Here's how the part is built. I have some questions about the finished solid (model axes, mm). Face numbers are marked on the shaded views. A direction names the side the tool comes from. Give positions to 0.01 mm unless a question says otherwise; leave off trailing zeros. Answer as CSV lines item,"result". Start each with the question number.
Item 1: Will these pins go through, and if not, where does the flat tip stop? P1, Ø5, axis at x = 19.5, z = 3, coming from the -Y side; P2, Ø6, axis at x = 6.5, z = 2, coming from the -Y side; P3, Ø3, axis at x = 17.5, z = 7.5, coming from the +Y side; P4, Ø6, axis at x = 25, y = 100, coming from the +Z side.
Item 2: If I drill on line 1 along X through (y, z) = (75.5, 7.5); line 2 along X through (y, z) = (86, 7.5); line 3 along Y through (x, z) = (34.5, 7), over which ranges is the centre line in solid material (lowest first)? Write a range as from..to.
Item 3: For the marked faces 3 and 4, which set-ups out of +Z, -Z, +X, -X, +Y, -Y let a thin tool reach every point of the face, with its end or its side?
Item 4: If we mould it in two halves opening along X, with no side actions, what happens to the marked faces 1 and 2? For each: released by +X, released by -X, zero draft, split by the parting line, or undercut.
Item 5: I want a section at A-A on z = 3.75. Give the number of separate pieces and of enclosed holes in the cut face, plus the area to 3 significant figures.
from build123d import *

# Parameters (mm, degrees)
SKETCH1_R           = 5
BOSS_EXTRUDE1_DEPTH = 10
CUT_EXTRUDE2_DEPTH  = 10
FILLET1_R           = 2
FILLET2_R           = 2


with BuildPart() as part:
    # Sketch1 → Boss-Extrude1 (new body)
    # profile 1 of 2: a face of its own
    with BuildSketch(Plane.XY):
        with BuildLine():
            Line((0, 0), (0, 100))
            ThreePointArc((0, 100), (25, 125), (50, 100))
            Line((50, 100), (50, 0))
            ThreePointArc((50, 0), (25, -25), (0, 0))
        make_face()
        with BuildLine():
            ThreePointArc((15, 0), (25, -10), (35, 0))
            Line((35, 0), (35, 100))
            ThreePointArc((35, 100), (25, 110), (15, 100))
            Line((15, 100), (15, 0))
        make_face(mode=Mode.SUBTRACT)
    # profile 2 of 2: a face of its own
    with BuildSketch(Plane.XY):
        with BuildLine():
            Line((15, 0), (15, 100))
            ThreePointArc((15, 100), (25, 110), (35, 100))
            Line((35, 100), (35, 0))
            ThreePointArc((35, 0), (25, -10), (15, 0))
        make_face()
        with Locations((25, 0)):
            Circle(SKETCH1_R, mode=Mode.SUBTRACT)
        with Locations((25, 100)):
            Circle(SKETCH1_R, mode=Mode.SUBTRACT)
    extrude(amount=BOSS_EXTRUDE1_DEPTH)

    # Sketch2 → Cut-Extrude2 (cut)
    with BuildSketch(Plane.XY.offset(10)):
        with BuildLine():
            Line((25.064971157, 89.343145751), (10, 89.343145751))
            Line((10, 89.343145751), (10, 70.656854249))
            Line((10, 70.656854249), (26.125631329, 86.782485579))
            ThreePointArc((26.125631329, 86.782485579), (26.450790456, 88.417170899), (25.064971157, 89.343145751))
        make_face()
        with BuildLine():
            Line((40, 69), (40, 89.343145751))
            Line((40, 89.343145751), (22.217514421, 71.560660172))
            ThreePointArc((22.217514421, 71.560660172), (21.892355294, 69.925974851), (23.278174593, 69))
            Line((23.278174593, 69), (40, 69))
        make_face()
        with BuildLine():
            Line((26.721825407, 61), (10, 61))
            Line((10, 61), (10, 40.65685425))
            Line((10, 40.65685425), (22.171572875, 52.828427125))
            Line((22.171572875, 52.828427125), (27.782485579, 58.439339828))
            ThreePointArc((27.782485579, 58.439339828), (28.107644706, 60.074025149), (26.721825407, 61))
        make_face()
        with BuildLine():
            Line((40, 39), (40, 59.343145751))
            Line((40, 59.343145751), (27.828427125, 47.171572875))
            Line((27.828427125, 47.171572875), (22.217514421, 41.560660172))
            ThreePointArc((22.217514421, 41.560660172), (21.892355294, 39.925974852), (23.278174593, 39))
            Line((23.278174593, 39), (40, 39))
        make_face()
        with BuildLine():
            Line((26.721825408, 31.000000001), (10, 31.000000001))
            Line((10, 31.000000001), (10, 10.656854249))
            Line((10, 10.656854249), (27.782485579, 28.439339829))
            ThreePointArc((27.782485579, 28.439339829), (28.107644706, 30.074025149), (26.721825408, 31.000000001))
        make_face()
        with BuildLine():
            Line((40, 9), (40, 29.34314575))
            Line((40, 29.34314575), (22.217514422, 11.560660171))
            ThreePointArc((22.217514422, 11.560660171), (21.892355295, 9.925974851), (23.278174594, 9))
            Line((23.278174594, 9), (40, 9))
        make_face()
    extrude(amount=-CUT_EXTRUDE2_DEPTH, mode=Mode.SUBTRACT)

    # Fillet1
    fillet1_edges = [part.edges().sort_by_distance(p)[0] for p in [
        (10, 10.656854249, 5),
        (10, 31.000000001, 5),
        (40, 59.343145751, 5),
        (40, 39, 5),
        (10, 40.65685425, 5),
        (10, 61, 5),
        (40, 89.343145751, 5),
        (40, 69, 5),
        (40, 29.34314575, 5),
        (40, 9, 5),
        (10, 70.656854249, 5),
        (10, 89.343145751, 5),
    ]]
    fillet(fillet1_edges, radius=FILLET1_R)

    # Fillet2
    fillet2_edges = [part.edges().sort_by_distance(p)[0] for p in [
        (25, -25, 0),
        (0, 50, 0),
        (25, -25, 10),
        (50, 50, 10),
        (25, 125, 10),
        (0, 50, 10),
        (25, 125, 0),
        (50, 50, 0),
    ]]
    fillet(fillet2_edges, radius=FILLET2_R)


solid = part.part
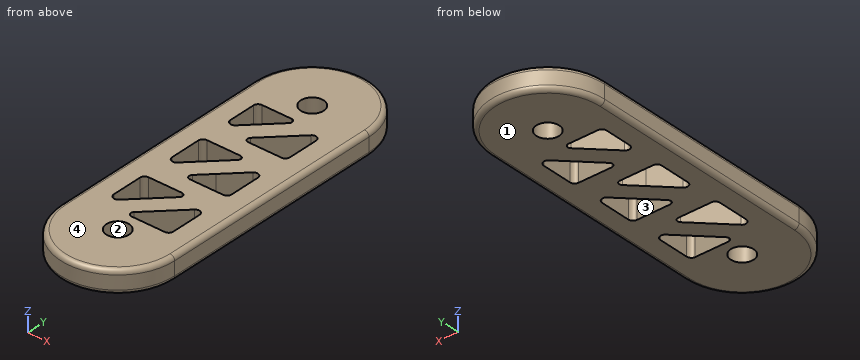
Result:
1,P1,"y = -24.82"
1,P2,"y = -19.62"
1,P3,"y = 124.27"
1,P4,"through"
2,line 1,"0..10, 14.84..26.16, 40..50"
2,line 2,"0..10, 25.34..36.66, 39.34..50"
2,line 3,"-23.12..9, 23.84..39, 53.84..69, 83.84..123.12"
3,face 3,"+Z, -Z"
3,face 4,"+Z, +X, -X, +Y, -Y"
4,face 1,"zero draft"
4,face 2,"undercut"
5,separate pieces,"1"
5,enclosed holes,"8"
5,area,"5,650 mm^2"
